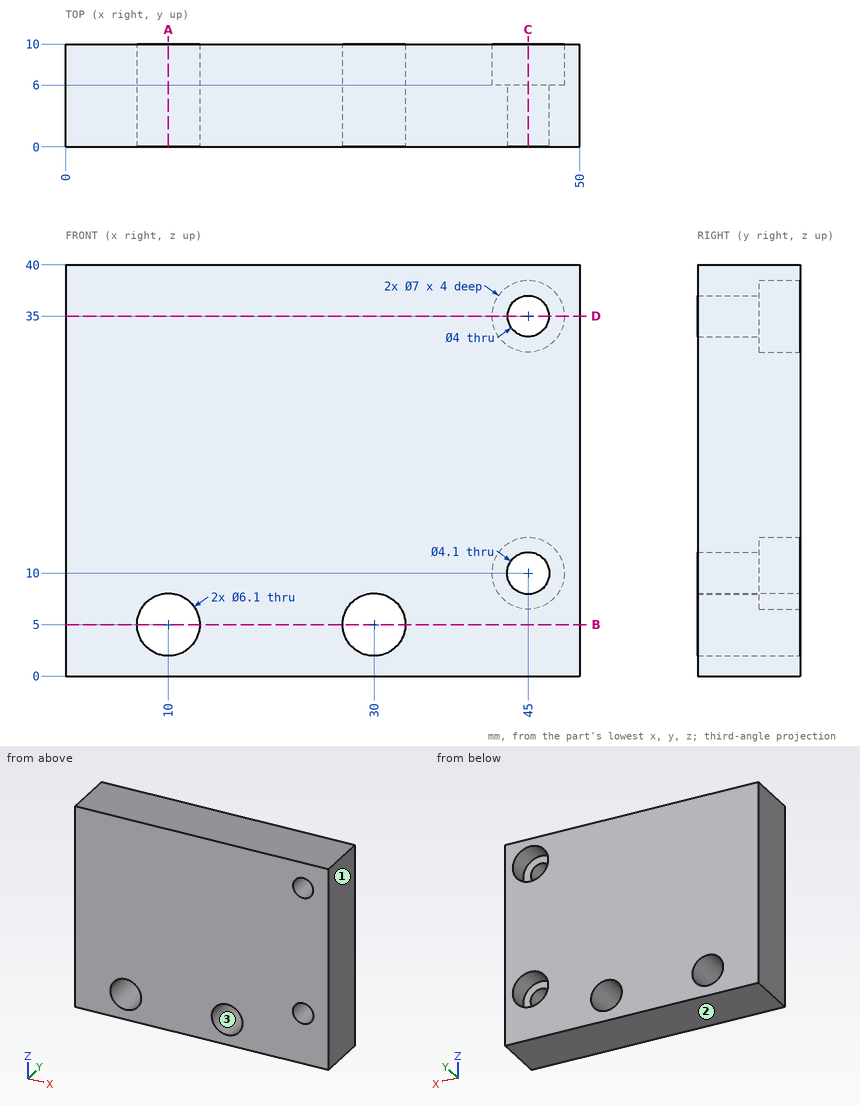
The drawing under review shows one solid part. Ordinate dimensions are in mm from its lowest x, y, z. Give positions to 0.01 mm unless a question says otherwise; leave off trailing zeros. Write each loop counter-clockwise with the first axis right and the second up, starting at its lowest first coordinate (ties: lowest second). Pieces come first, ordered by that corner, then holes. Notation, with made-up numbers: M 8.5,-37 L 54.5,-37 A26 ccw 54.5,-18 Z; hole C 2.25,53.5 d7. An arc over 180 degrees is marked long. Write each question's results on one line, items separated by ' | '. Start each with the question number.
1. We need section A-A (x = 10). Write out the cut boundary in (y, z), and give its area (3 significant figures).
2. Mouldability with a two-part tool opening along X and no side actions: class the marked faces 1, 2 and 3 as released by +X, released by -X, zero draft, split by the parting line, or undercut.
3. For probe 1 along X at (y, z) = (5, 5); probe 2 along Z at (x, y) = (45, 3.65); probe 3 along Z at (x, y) = (45, 7.95), list the stretches that pass through material, from the lowest coordinate up. Write a range as [from, to].
4. We need section C-C (x = 45). Write out the cut boundary in (y, z).
5. We need section B-B (z = 5). Write out the cut boundary in (x, y).
6. Insertion check: pin 1 Ø5.5 at (x, z) = (45, 35) entering from +Y. The pin has a flat end and moves straight along its axis. Give the tip position at first contact, or say it passes through.
7. We need section D-D (z = 35). Write out the cut boundary in (x, y), and give its area (3 significant figures).
Results found:
1) outline: M 0,0 L 10,0 L 10,1.95 L 0,1.95 Z; M 0,8.05 L 10,8.05 L 10,40 L 0,40 Z | area: 339 mm^2
2) face 1: released by +X | face 2: zero draft | face 3: undercut
3) probe 1: x = [0, 6.95], [13.05, 26.95], [33.05, 50] | probe 2: z = [0, 7.95], [12.05, 33], [37, 40] | probe 3: z = [0, 6.5], [13.5, 31.5], [38.5, 40]
4) outline: M 0,0 L 10,0 L 10,6.5 L 6,6.5 L 6,7.95 L 0,7.95 Z; M 0,12.05 L 6,12.05 L 6,13.5 L 10,13.5 L 10,31.5 L 6,31.5 L 6,33 L 0,33 Z; M 0,37 L 6,37 L 6,38.5 L 10,38.5 L 10,40 L 0,40 Z
5) outline: M 0,0 L 6.95,0 L 6.95,10 L 0,10 Z; M 13.05,0 L 26.95,0 L 26.95,10 L 13.05,10 Z; M 33.05,0 L 50,0 L 50,10 L 33.05,10 Z
6) pin 1: stops at y = 6
7) outline: M 0,0 L 43,0 L 43,6 L 41.5,6 L 41.5,10 L 0,10 Z; M 47,0 L 50,0 L 50,10 L 48.5,10 L 48.5,6 L 47,6 Z | area: 448 mm^2
